Check sheet for the modelled part. Datum: model origin and axes. Units: mm. A direction names the side the tool comes from. Give positions to 0.01 mm unless a question says otherwise; leave off trailing zeros. Write each loop counter-clockwise with the first axis right and the second up, starting at its lowest first coordinate (ties: lowest second). Pieces come first, ordered by that corner, then holes. Notation, with made-up numbers: (65, 58.25) -> (81, 58.25) arc R11 cw to (81, 73.25) -> close; hole circle Ø8 at (-21.75, -10.75). An arc over 180 degrees is marked (long way). Use a Markdown table: item, result. Add a question column.
1. Scan lines: probe 1 along Z at (x, y) = (-18.5, 34.5); probe 2 along X at (y, z) = (-82, 6.5). Record each from-to range of solid material in increasing order. Write a range as [from, to].
2. Gauge pin test, flat end, axial feed: P1, Ø1.5, axis at y = 46, z = 8.5, coming from the -X side. Record the tip position at first contact, or that the pin passes through.
3. Cross-section at B-B (z = 8). Enter the section's corners in (x, y).
4. Set-up check for faces 1 (the flat face through (-10, 1, 5.471)), 2 (the flat face through (-26.047, -1, -3)): record each of +Z, -Z, +X, -X, +Y, -Y from which the full face is reachable in a straight line by a thin tool's end or side.
5. Cross-section at C-C (x = -22). Enter the section's corners in (y, z).
6. Cross-section at A-A (y = 36.5). Enter the section's corners in (x, z).
from build123d import *

# Parameters (mm, degrees)
F0_W     = 52.0943142474
F0_H     = 21.1019426874
F1_DEPTH = 105.537
F2_W     = 31.9535313174
F2_H     = 211.074
F3_DEPTH = 5.08


with BuildPart() as f1:
    # F0 (on Front) → F1 (new body, symmetric)
    with BuildSketch(Plane.XZ):
        Rectangle(F0_W, F0_H)
    extrude(amount=F1_DEPTH, both=True)

    # F2 (on face) → F3 (cut)
    with BuildSketch(Plane.XY.offset(10.5509713437)):
        with Locations((-10.070391465, 0)):
            Rectangle(F2_W, F2_H)
    extrude(amount=-F3_DEPTH, mode=Mode.SUBTRACT)


solid = f1.part
Worked answers:
| question | item | result |
|---|---|---|
| 1 | probe 1 | z = [-10.55, 5.47] |
| 1 | probe 2 | x = [5.91, 26.05] |
| 2 | P1 | stops at x = 5.91 |
| 3 | outline | (5.91, -105.54) -> (26.05, -105.54) -> (26.05, 105.54) -> (5.91, 105.54) -> close |
| 4 | face 1 | +Z, -X, +Y, -Y |
| 4 | face 2 | +Z, -Z, -X, +Y, -Y |
| 5 | outline | (-105.54, -10.55) -> (105.54, -10.55) -> (105.54, 5.47) -> (-105.54, 5.47) -> close |
| 6 | outline | (-26.05, -10.55) -> (26.05, -10.55) -> (26.05, 10.55) -> (5.91, 10.55) -> (5.91, 5.47) -> (-26.05, 5.47) -> close |
